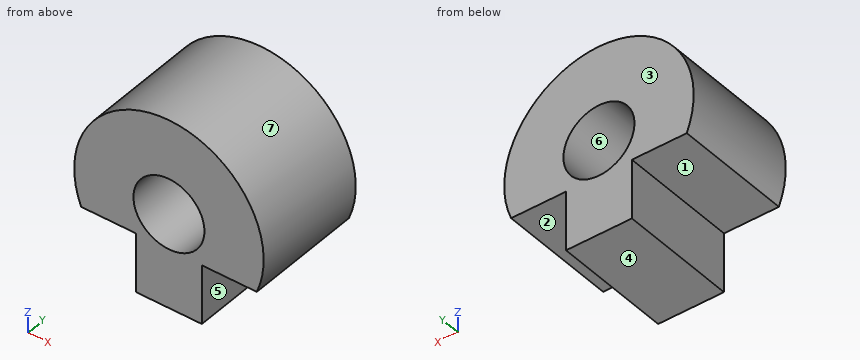
from build123d import *

# Parameters (mm, degrees)
SKETCH1_R           = 1.905
BOSS_EXTRUDE1_DEPTH = 6.35


with BuildPart() as part:
    # Sketch1 → Boss-Extrude1 (new body)
    with BuildSketch(Plane(origin=(0, 0, 0), x_dir=(1, 0, 0), z_dir=(0, 1, 0))):
        with BuildLine():
            Line((-1.7653, 1.905), (-1.7653, 5.08))
            Line((-1.7653, 5.08), (1.7653, 5.08))
            Line((1.7653, 5.08), (1.7653, 1.905))
            Line((1.7653, 1.905), (4.709286039, 1.905))
            ThreePointArc((4.709286039, 1.905), (0, -5.08), (-4.709286039, 1.905))
            Line((-4.709286039, 1.905), (-1.7653, 1.905))
        make_face()
        Circle(SKETCH1_R, mode=Mode.SUBTRACT)
    extrude(amount=BOSS_EXTRUDE1_DEPTH)


solid = part.part
Read the model definition and answer for the solid it produces. Units are mm, in the model's axes. Face numbers are marked on the shaded views. A direction names the side the tool comes from. Round coordinates to 2 decimals unless told otherwise and drop trailing zeros. Order: outer loops, then holes, each group sorted by start corner. A loop starts at its lowest first (then second) coordinate and runs counter-clockwise, first axis right, second up.
1) Straight lines are drawn through the part: L1, parallel to X at y = 5.25, z = 0 (3 decimals); L2, parallel to X at y = 4, z = 2. For each, find the intervals that lie inside material, in ascending order.
2) The part is cut by section D-D on z = -2.5. Write down the section's boundary in (x, y).
3) Flat-ended cylindrical pins translate along their axes: pin 1 (2 mm diameter, centred on x = -4, y = 1.5, fed in from +Z); pin 2 (3 mm diameter, centred on x = 2.5, y = 4, fed in from +Z); pin 3 (1 mm diameter, centred on y = 0.5, z = 2.5, fed in from +X). Find the tip coordinate at first contact, or state that the pin passes through.
4) The part is cut by section B-B on x = 0. Write down the section's boundary in (y, z) (3 decimals).
5) The mould has two halves that part along X. Classify the marked faces 4, 5, 6 and 7: released by +X, released by -X, zero draft, split by the parting line, or undercut.
6) The part is cut by section C-C on z = 0. Write down the section's boundary in (x, y) (3 decimals).
7) The part is cut by section A-A on y = 4.5. Write down the section's boundary in (x, z) (3 decimals).
8) For the marked faces 1, 2 and 3, determine the directions among +Z, -Z, +X, -X, +Y, -Y from which every point of the face is accessible in a straight line to the end or side of a thin tool.
Resolved:
1. L1: x = -5.08 to -1.905, 1.905 to 5.08
1. L2: x = -4.67 to 4.67
2. outline: (-1.77, 0) - (1.77, 0) - (1.77, 6.35) - (-1.77, 6.35) - close
3. pin 1: stops at z = 4.1
3. pin 2: stops at z = 4.98
3. pin 3: stops at x = 4.67
4. outline: (0, -5.08) - (6.35, -5.08) - (6.35, -1.905) - (0, -1.905) - close; (0, 1.905) - (6.35, 1.905) - (6.35, 5.08) - (0, 5.08) - close
5. face 4: zero draft
5. face 5: released by +X
5. face 6: undercut
5. face 7: split by the parting line
6. outline: (-5.08, 0) - (-1.905, 0) - (-1.905, 6.35) - (-5.08, 6.35) - close; (1.905, 0) - (5.08, 0) - (5.08, 6.35) - (1.905, 6.35) - close
7. outline: (-4.709, -1.905) - (-1.765, -1.905) - (-1.765, -5.08) - (1.765, -5.08) - (1.765, -1.905) - (4.709, -1.905) arc R5.08 ccw (long way) to start; hole circle Ø3.81 at (0, 0)
8. face 1: -Z, -X, +Y, -Y
8. face 2: -Z, +X, +Y, -Y
8. face 3: +Z, -Z, +X, -X, +Y
